```python
from build123d import *

# Parameters (mm, degrees)
F0_R      = 52.5
F1_DEPTH  = 3
F2_R      = 43
F3_DEPTH  = 22
F4_R      = 8.5
F5_DEPTH  = 11
F6_R      = 5.5
F7_DEPTH  = 11.001
F8_SIZE2  = 1.5
F8_SIZE   = 10
F9_R      = 4
F10_DEPTH = 50


with BuildPart() as f1:
    # F0 (on Front) → F1 (new body)
    with BuildSketch(Plane.XZ):
        Circle(F0_R)
    extrude(amount=F1_DEPTH)

    # F2 (on face) → F3 (join)
    with BuildSketch(Plane.XZ.offset(3)):
        Circle(F2_R)
    extrude(amount=-F3_DEPTH)

    # F4 (on face) → F5 (cut)
    with BuildSketch(Plane.XZ.offset(3)):
        with Locations((-21.25, 0)):
            Circle(F4_R)
    extrude(amount=-F5_DEPTH, mode=Mode.SUBTRACT)

    # F6 (on face) → F7 (cut, through all)
    with BuildSketch(Plane.XZ.offset(-8)):
        with Locations((-21.25, 0)):
            Circle(F6_R)
    extrude(amount=-F7_DEPTH, mode=Mode.SUBTRACT)

    # F8
    f8_edges = [f1.edges().sort_by_distance(p)[0] for p in [
        (-52.5, -3, 0),
    ]]
    f8_side = f1.faces().sort_by_distance((0.572024, -3, 0))[0]
    chamfer(f8_edges, length=F8_SIZE, length2=F8_SIZE2, reference=f8_side)

    # F9 (on Top) → F10 (cut, symmetric)
    with BuildSketch(Plane.XY):
        with Locations((0, 7)):
            Circle(F9_R)
    extrude(amount=F10_DEPTH, both=True, mode=Mode.SUBTRACT)


solid = f1.part
```
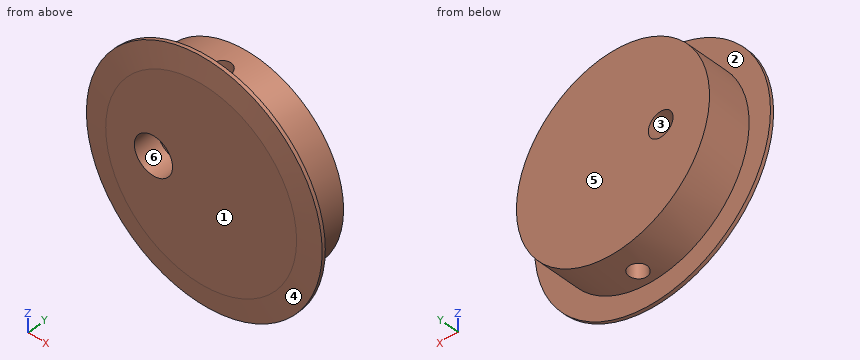
Could you check a few things on this model? Use its own coordinates, in mm. Face numbers are marked on the shaded views. A direction names the side the tool comes from. Round coordinates to 2 decimals unless told otherwise and drop trailing zeros. Write each loop counter-clockwise with the first axis right and the second up, starting at its lowest first coordinate (ties: lowest second). Pieces come first, ordered by that corner, then holes. Notation, with made-up numbers: M 52.25,-10 L 90.25,-10 A24 cw 90.25,29 Z; hole C 4,-22.75 d4. An arc over 180 degrees is marked long. Answer in a Markdown table with one row per item. Add a question column.
Q1. If we mould it in two halves opening along Z, with no side actions, what happens to the marked faces 3, 4, 5 and 6? For each: +Z half, -Z half, draft (parallel to the pull), parting line (faces both ways), or undercut.
Q2. On a 3-axis mill with a long thin cutter (end or side, diameter ignored), from which of +Z, -Z, +X, -X, +Y, -Y can I reach the whole of each face in a straight line? I mean the marked faces 1 and 2. Say none if no direction works.
Q3. If I drill on line 1 (Y direction, x = 0, z = 9); line 2 (X direction, y = 8, z = -23); line 3 (X direction, y = 1.25, z = 3.5), over which ranges is the centre line in solid material (lowest first)? Write a range as from..to.
Q4. Will these pins go through, and if not, where does the flat tip stop? pin 1 Ø1.5 at (x, y) = (32.5, 14) entering from +Z; pin 2 Ø1 at (y, z) = (10.5, -10.5) entering from -X; pin 3 Ø6 at (x, y) = (-41, 9.5) entering from -Z; pin 4 Ø6.5 at (x, y) = (0, 7) entering from -Z.
Q5. Imagine slicing it at A-A (x = 0). Please give me the cut outline in (y, z), then the cut area to 3 significant figures.
Q6. Imagine slicing it at B-B (z = 0). Please give me the cut outline in (x, y), then the cut area to 3 significant figures.
Values:
| question | item | result |
|---|---|---|
| 1 | face 3 | undercut |
| 1 | face 4 | parting line |
| 1 | face 5 | draft |
| 1 | face 6 | undercut |
| 2 | face 1 | +Z, -Z, +X, -X, -Y |
| 2 | face 2 | +Y |
| 3 | line 1 | -3..3, 11..19 |
| 3 | line 2 | -36.33..-3.87, 3.87..36.33 |
| 3 | line 3 | -42.86..-29, -13.5..42.86 |
| 4 | pin 1 | z = 29 |
| 4 | pin 2 | x = -41.82 |
| 4 | pin 3 | z = -20.12 |
| 4 | pin 4 | through |
| 5 | outline | M -3,-42.5 L -1.5,-52.5 L 0,-52.5 L 0,-43 L 3,-43 L 3,43 L 0,43 L 0,52.5 L -1.5,52.5 L -3,42.5 Z; M 11,-43 L 19,-43 L 19,43 L 11,43 Z |
| 5 | area | 1,250 mm^2 |
| 6 | outline | M -52.5,-1.5 L -42.5,-3 L -29.75,-3 L -29.75,8 L -26.75,8 L -26.75,19 L -43,19 L -43,0 L -52.5,0 Z; M -15.75,8 L -12.75,8 L -12.75,-3 L 42.5,-3 L 52.5,-1.5 L 52.5,0 L 43,0 L 43,19 L -15.75,19 Z; hole C 0,7 d8 |
| 6 | area | 1,580 mm^2 |
